Can you work these out from the model? Positions are in its coordinate system, mm. Coordinates: 2 decimals unless noted, no trailing zeros. Loops run counter-clockwise (first coordinate to the right, second up) from the corner with the lowest first, then second, coordinate; pieces in that order, holes last.
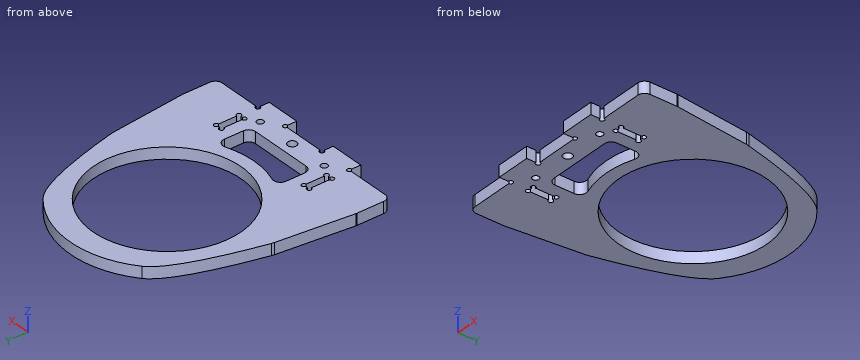
```python
from build123d import *

# Parameters (mm, degrees)
SKETCH_1_R          = 32.5
EXTRUDE_1_DEPTH     = 5
SKETCH_2_W          = 15
SKETCH_2_H          = 5
EXTRUDE_2_DEPTH     = 5
SKETCH_3_R          = 1
CUT_EXTRUDE_1_DEPTH = 114.081828779
SKETCH_4_R          = 1.95
SKETCH_4_R_2        = 1.45
CUT_EXTRUDE_2_DEPTH = 114.081828779
FILLET_1_R          = 3
SKETCH_5_W          = 2.9
SKETCH_5_H          = 10
CUT_EXTRUDE_3_DEPTH = 114.081828779
SKETCH_6_R          = 1
CUT_EXTRUDE_4_DEPTH = 114.081828779
CUT_EXTRUDE_5_DEPTH = 114.081828779
FILLET_3_R          = 10
FILLET_4_R          = 3


with BuildPart() as part:
    # Sketch 1 → Extrude 1 (new body)
    with BuildSketch(Plane.XY):
        with BuildLine():
            Line((-42.263952975, 64.473061473), (-47.5, 15))
            Line((-47.5, 15), (-47.5, 0))
            Line((-47.5, 0), (47.5, 0))
            Line((47.5, 0), (47.5, 15))
            Line((47.5, 15), (42.263952975, 64.473061473))
            ThreePointArc((42.263952975, 64.473061473), (0, 102.5), (-42.263952975, 64.473061473))
        make_face()
        with Locations((0, 60)):
            Circle(SKETCH_1_R, mode=Mode.SUBTRACT)
    extrude(amount=EXTRUDE_1_DEPTH)

    # Sketch 2 → Extrude 2 (add)
    with BuildSketch(Plane.XY.offset(5)):
        with Locations((-17.5, -2.5)):
            Rectangle(SKETCH_2_W, SKETCH_2_H)
        with Locations((17.5, -2.5)):
            Rectangle(SKETCH_2_W, SKETCH_2_H)
    extrude(amount=-EXTRUDE_2_DEPTH)

    # Sketch 3 → Cut-Extrude 1 (cut, through all)
    with BuildSketch(Plane.XY.offset(5)):
        with Locations((-25, 0)):
            Circle(SKETCH_3_R)
        with Locations((-10, 0)):
            Circle(SKETCH_3_R)
        with Locations((10, 0)):
            Circle(SKETCH_3_R)
        with Locations((25, 0)):
            Circle(SKETCH_3_R)
    extrude(amount=-CUT_EXTRUDE_1_DEPTH, mode=Mode.SUBTRACT)

    # Sketch 4 → Cut-Extrude 2 (cut, through all)
    with BuildSketch(Plane.XY.offset(5)):
        with Locations((0, 5)):
            Circle(SKETCH_4_R)
        with Locations((-17.5, 5)):
            Circle(SKETCH_4_R_2)
        with Locations((17.5, 5)):
            Circle(SKETCH_4_R_2)
    extrude(amount=-CUT_EXTRUDE_2_DEPTH, mode=Mode.SUBTRACT)

    # Fillet 1
    fillet_1_edges = [part.edges().sort_by_distance(p)[0] for p in [
        (47.5, 15, 2.5),
        (47.5, 0, 2.5),
        (-47.5, 0, 2.5),
        (-47.5, 15, 2.5),
    ]]
    fillet(fillet_1_edges, radius=FILLET_1_R)

    # Sketch 5 → Cut-Extrude 3 (cut, through all)
    with BuildSketch(Plane.XY.offset(5)):
        with Locations((-23.95, 13)):
            Rectangle(SKETCH_5_W, SKETCH_5_H)
        with Locations((23.95, 13)):
            Rectangle(SKETCH_5_W, SKETCH_5_H)
    extrude(amount=-CUT_EXTRUDE_3_DEPTH, mode=Mode.SUBTRACT)

    # Sketch 6 → Cut-Extrude 4 (cut, through all)
    with BuildSketch(Plane.XY.offset(5)):
        with Locations((-25.4, 18)):
            Circle(SKETCH_6_R)
        with Locations((-22.5, 18)):
            Circle(SKETCH_6_R)
        with Locations((-22.5, 8)):
            Circle(SKETCH_6_R)
        with Locations((-25.4, 8)):
            Circle(SKETCH_6_R)
        with Locations((22.5, 18)):
            Circle(SKETCH_6_R)
        with Locations((25.4, 18)):
            Circle(SKETCH_6_R)
        with Locations((25.4, 8)):
            Circle(SKETCH_6_R)
        with Locations((22.5, 8)):
            Circle(SKETCH_6_R)
    extrude(amount=-CUT_EXTRUDE_4_DEPTH, mode=Mode.SUBTRACT)

    # Sketch 7 → Cut-Extrude 5 (cut, through all)
    with BuildSketch(Plane.XY.offset(5)):
        with BuildLine():
            Line((-16.805922522, 25.815370212), (-16.805922522, 9.999999776))
            Line((-16.805922522, 9.999999776), (16.805922522, 9.999999776))
            Line((16.805922522, 9.999999776), (16.805922522, 25.815370212))
            ThreePointArc((16.805922522, 25.815370212), (0, 21.907639276), (-16.805922522, 25.815370212))
        make_face()
        with BuildLine():
            Line((-46.54378056, 48.762700401), (-46.54378056, 92.803684493))
            Line((-46.54378056, 92.803684493), (-27.021626223, 92.803684493))
            add(Edge.make_bspline(
                [(-27.021626223, 92.803684493), (-35.335790396, 85.954995386), (-43.926679859, 48.762700401)],
                knots=[0, 0, 0, 1, 1, 1], degree=2))
            Line((-43.926679859, 48.762700401), (-46.54378056, 48.762700401))
        make_face()
        with BuildLine():
            Line((46.54378056, 92.803684493), (27.021626223, 92.803684493))
            add(Edge.make_bspline(
                [(27.021626223, 92.803684493), (35.335790396, 85.954995386), (43.926679859, 48.762700401)],
                knots=[0, 0, 0, 1, 1, 1], degree=2))
            Line((43.926679859, 48.762700401), (46.54378056, 48.762700401))
            Line((46.54378056, 48.762700401), (46.54378056, 92.803684493))
        make_face()
    extrude(amount=-CUT_EXTRUDE_5_DEPTH, mode=Mode.SUBTRACT)

    # Fillet 3
    fillet_3_edges = [part.edges().sort_by_distance(p)[0] for p in [
        (-43.926679859, 48.762700401, 2.5),
        (43.926679859, 48.762700401, 2.5),
    ]]
    fillet(fillet_3_edges, radius=FILLET_3_R)

    # Fillet 4
    fillet_4_edges = [part.edges().sort_by_distance(p)[0] for p in [
        (-16.805922522, 25.815370212, 2.5),
        (16.805922522, 25.815370212, 2.5),
        (16.805922522, 9.999999776, 2.5),
        (-16.805922522, 9.999999776, 2.5),
    ]]
    fillet(fillet_4_edges, radius=FILLET_4_R)


solid = part.part
```
(1) I want a section at A-A on x = 6. Write out the boundary of the cut face in (y, z).
Check values:
outline: (0, 0) - (10, 0) - (10, 5) - (0, 5) - close; (22.38, 0) - (28.06, 0) - (28.06, 5) - (22.38, 5) - close; (91.94, 0) - (102.07, 0) - (102.07, 5) - (91.94, 5) - close
(2) I want a section at B-B on y = 46. Write out the boundary of the cut face in (x, z).
Check values:
outline: (-44.22, 0) - (-29.33, 0) - (-29.33, 5) - (-44.22, 5) - close; (29.33, 0) - (44.22, 0) - (44.22, 5) - (29.33, 5) - close
(3) I want a section at C-C on z = 3. State how many separate pieces and enclosed holes the cut face has, then the cut area to 3 significant figures.
Check values:
separate pieces: 1
enclosed holes: 7
area: 4,450 mm2
(4) I'm going to push flat-ended pins straight in: pin 1 (1 mm diameter, centred on y = 16.5, z = 4, fed in from -X); pin 2 (2.5 mm diameter, centred on y = 17, z = 2, fed in from +X); pin 3 (1.6 mm diameter, centred on x = -25.4, y = 8, fed in from +Z); pin 4 (3 mm diameter, centred on y = 29.5, z = 0.5, fed in from -X). Where does each tip first touch, or does it pass through?
Check values:
pin 1: stops at x = -47.39
pin 2: stops at x = 47.42
pin 3: passes through
pin 4: stops at x = -46.12
(5) If I drill on probe 1 along Y at (x, z) = (-12, 4.2); probe 2 along Y at (x, z) = (2.5, 3.3); probe 3 along X at (y, z) = (68, 1.3), over which ranges is the centre line in solid material (lowest first)?
Check values:
probe 1: y = -5 to 10, 23.85 to 29.8, 90.2 to 100.77
probe 2: y = 0 to 10, 21.99 to 27.6, 92.4 to 102.43
probe 3: x = -38.9 to -31.5, 31.5 to 38.9
